Part model, mm, in its own coordinate system. Face numbers are marked on the shaded views. A direction names the side the tool comes from. Give positions to 0.01 mm unless a question says otherwise; leave off trailing zeros. Write each loop counter-clockwise with the first axis right and the second up, starting at its lowest first coordinate (ties: lowest second). Pieces come first, ordered by that corner, then holes. Notation, with made-up numbers: M -22.75,2 L 35.25,2 A22 cw 35.25,29 Z; hole C -40,4.25 d3. An arc over 180 degrees is marked long. Use a Markdown table: item, result.
```python
from build123d import *

# Parameters (mm, degrees)
SKETCH_W        = 160.02
SKETCH_H        = 160.02
PAD_DEPTH       = 5.08
SKETCH001_W     = 2.032
SKETCH001_H     = 160.02
PAD001_DEPTH    = 1.016
SKETCH002_W     = 160.02
SKETCH002_H     = 2.032
PAD002_DEPTH    = 1.016
SKETCH003_W     = 6.35
SKETCH003_H     = 12.7
PAD003_DEPTH    = 10.16
SKETCH004_R     = 2.032
POCKET_DEPTH    = 12.7
PAD004_DEPTH    = 160.02
PAD005_DEPTH    = 160.02
SKETCH007_R     = 5.2705
POCKET001_DEPTH = 7.366
SKETCH008_R     = 2.286
POCKET002_DEPTH = 12.7
SKETCH009_R     = 5.2705
POCKET003_DEPTH = 7.366
SKETCH010_R     = 2.286
POCKET004_DEPTH = 12.7
SKETCH011_R     = 5.2705
POCKET005_DEPTH = 7.366
SKETCH012_R     = 5.2705
POCKET006_DEPTH = 7.366
SKETCH013_R     = 2.286
POCKET007_DEPTH = 12.7
SKETCH014_R     = 2.286
POCKET008_DEPTH = 12.7
SKETCH015_W     = 6.35
SKETCH015_H     = 12.7
PAD006_DEPTH    = 10.16
SKETCH016_R     = 2.032
POCKET009_DEPTH = 12.7


with BuildPart() as part:
    # Sketch → Pad (new body)
    with BuildSketch(Plane.XY):
        with Locations((-8.701914, -21.351993)):
            Rectangle(SKETCH_W, SKETCH_H)
    extrude(amount=PAD_DEPTH)

    # Sketch001 (on Face6 of Pad) → Pad001 (join)
    with BuildSketch(Plane.XY.offset(5.08)):
        with Locations((-62.295914, -21.351993)):
            Rectangle(SKETCH001_W, SKETCH001_H)
        with Locations((44.892086, -21.351993)):
            Rectangle(SKETCH001_W, SKETCH001_H)
        with Locations((-13.527914, -21.351993)):
            Rectangle(SKETCH001_W, SKETCH001_H)
        with Locations((-3.875914, -21.351993)):
            Rectangle(SKETCH001_W, SKETCH001_H)
    extrude(amount=PAD001_DEPTH)

    # Sketch002 (on Face9 of Pad001) → Pad002 (join)
    with BuildSketch(Plane.XY.offset(5.08)):
        with Locations((-8.701914, 32.242007)):
            Rectangle(SKETCH002_W, SKETCH002_H)
        with Locations((-8.701914, -16.525993)):
            Rectangle(SKETCH002_W, SKETCH002_H)
        with Locations((-8.701914, -26.177993)):
            Rectangle(SKETCH002_W, SKETCH002_H)
        with Locations((-8.701914, -74.945993)):
            Rectangle(SKETCH002_W, SKETCH002_H)
    extrude(amount=PAD002_DEPTH)

    # Sketch003 (on Face164 of Pad002) → Pad003 (join)
    with BuildSketch(Plane.XY.offset(5.08)):
        with Locations((-56.961914, -44.211993)):
            Rectangle(SKETCH003_W, SKETCH003_H)
        with Locations((39.558086, -44.211993)):
            Rectangle(SKETCH003_W, SKETCH003_H)
    extrude(amount=PAD003_DEPTH)

    # Sketch004 (on Face174 of Pad003) → Pocket (cut)
    with BuildSketch(Plane.XZ.offset(50.561993)):
        with Locations((39.558086, 11.43)):
            Circle(SKETCH004_R)
        with Locations((-56.961914, 11.43)):
            Circle(SKETCH004_R)
    extrude(amount=-POCKET_DEPTH, mode=Mode.SUBTRACT)

    # Sketch005 (on Face14 of Pocket) → Pad004 (join)
    with BuildSketch(Plane.XZ.offset(101.361993)):
        Polygon((-88.711914, 5.08), (-88.711914, 22.86), (-84.901914, 22.86), (-76.011914, 8.89), (-76.011914, 5.08), align=None)
        Polygon((71.308086, 22.86), (67.498086, 22.86), (58.608086, 8.89), (58.608086, 5.08), (71.308086, 5.08), align=None)
    extrude(amount=-PAD004_DEPTH)

    # Sketch006 (on Face3 of Pad004) → Pad005 (join)
    with BuildSketch(Plane.YZ.offset(71.308086)):
        Polygon((-101.361993, 5.08), (-101.361993, 22.86), (-97.551993, 22.86), (-88.661993, 8.89), (-88.661993, 5.08), align=None)
        Polygon((58.658007, 5.08), (58.658007, 22.86), (54.848007, 22.86), (45.958007, 8.89), (45.958007, 5.08), align=None)
    extrude(amount=-PAD005_DEPTH)

    # Sketch007 (on Face66 of Pad005) → Pocket001 (cut)
    with BuildSketch(Plane(origin=(0, -88.661993, 0), x_dir=(-1, 0, 0), z_dir=(0, 1, 0))):
        with Locations((-39.558086, 15.24)):
            Circle(SKETCH007_R)
        with Locations((56.961914, 15.24)):
            Circle(SKETCH007_R)
        with Locations((8.701914, 15.24)):
            Circle(SKETCH007_R)
    extrude(amount=-POCKET001_DEPTH, mode=Mode.SUBTRACT)

    # Sketch008 (on Face66 of Pad005) → Pocket002 (cut)
    with BuildSketch(Plane(origin=(0, -88.661993, 0), x_dir=(-1, 0, 0), z_dir=(0, 1, 0))):
        with Locations((-39.558086, 15.24)):
            Circle(SKETCH008_R)
        with Locations((56.961914, 15.24)):
            Circle(SKETCH008_R)
        with Locations((8.701914, 15.24)):
            Circle(SKETCH008_R)
    extrude(amount=-POCKET002_DEPTH, mode=Mode.SUBTRACT)

    # Sketch009 (on Face53 of Pocket002) → Pocket003 (cut)
    with BuildSketch(Plane.YZ.offset(-76.011914)):
        with Locations((-69.611993, 15.24)):
            Circle(SKETCH009_R)
        with Locations((-21.351993, 15.24)):
            Circle(SKETCH009_R)
        with Locations((26.908007, 15.24)):
            Circle(SKETCH009_R)
    extrude(amount=-POCKET003_DEPTH, mode=Mode.SUBTRACT)

    # Sketch010 (on Face53 of Pocket003) → Pocket004 (cut)
    with BuildSketch(Plane.YZ.offset(-76.011914)):
        with Locations((-69.611993, 15.24)):
            Circle(SKETCH010_R)
        with Locations((-21.351993, 15.24)):
            Circle(SKETCH010_R)
        with Locations((26.908007, 15.24)):
            Circle(SKETCH010_R)
    extrude(amount=-POCKET004_DEPTH, mode=Mode.SUBTRACT)

    # Sketch011 (on Face54 of Pocket004) → Pocket005 (cut)
    with BuildSketch(Plane.XZ.offset(-45.958007)):
        with Locations((-56.961914, 15.24)):
            Circle(SKETCH011_R)
        with Locations((-8.701914, 15.24)):
            Circle(SKETCH011_R)
        with Locations((39.558086, 15.24)):
            Circle(SKETCH011_R)
    extrude(amount=-POCKET005_DEPTH, mode=Mode.SUBTRACT)

    # Sketch012 (on Face75 of Pocket005) → Pocket006 (cut)
    with BuildSketch(Plane(origin=(58.608086, 0, 0), x_dir=(0, -1, 0), z_dir=(-1, 0, 0))):
        with Locations((-26.908007, 15.24)):
            Circle(SKETCH012_R)
        with Locations((21.351993, 15.24)):
            Circle(SKETCH012_R)
        with Locations((69.611993, 15.24)):
            Circle(SKETCH012_R)
    extrude(amount=-POCKET006_DEPTH, mode=Mode.SUBTRACT)

    # Sketch013 (on Face75 of Pocket005) → Pocket007 (cut)
    with BuildSketch(Plane(origin=(58.608086, 0, 0), x_dir=(0, -1, 0), z_dir=(-1, 0, 0))):
        with Locations((-26.908007, 15.24)):
            Circle(SKETCH013_R)
        with Locations((21.351993, 15.24)):
            Circle(SKETCH013_R)
        with Locations((69.611993, 15.24)):
            Circle(SKETCH013_R)
    extrude(amount=-POCKET007_DEPTH, mode=Mode.SUBTRACT)

    # Sketch014 (on Face54 of Pocket004) → Pocket008 (cut)
    with BuildSketch(Plane.XZ.offset(-45.958007)):
        with Locations((-56.961914, 15.24)):
            Circle(SKETCH014_R)
        with Locations((-8.701914, 15.24)):
            Circle(SKETCH014_R)
        with Locations((39.558086, 15.24)):
            Circle(SKETCH014_R)
    extrude(amount=-POCKET008_DEPTH, mode=Mode.SUBTRACT)

    # Sketch015 (on Face164 of Pad002) → Pad006 (join)
    with BuildSketch(Plane.XY.offset(5.08)):
        with Locations((-56.961914, 1.508007)):
            Rectangle(SKETCH015_W, SKETCH015_H)
        with Locations((39.558086, 1.508007)):
            Rectangle(SKETCH015_W, SKETCH015_H)
    extrude(amount=PAD006_DEPTH)

    # Sketch016 (on Face254 of Pad006) → Pocket009 (cut)
    with BuildSketch(Plane(origin=(0, 7.858007, 0), x_dir=(-1, 0, 0), z_dir=(0, 1, 0))):
        with Locations((56.961914, 11.176)):
            Circle(SKETCH016_R)
        with Locations((-39.558086, 11.176)):
            Circle(SKETCH016_R)
    extrude(amount=-POCKET009_DEPTH, mode=Mode.SUBTRACT)


solid = part.part
```
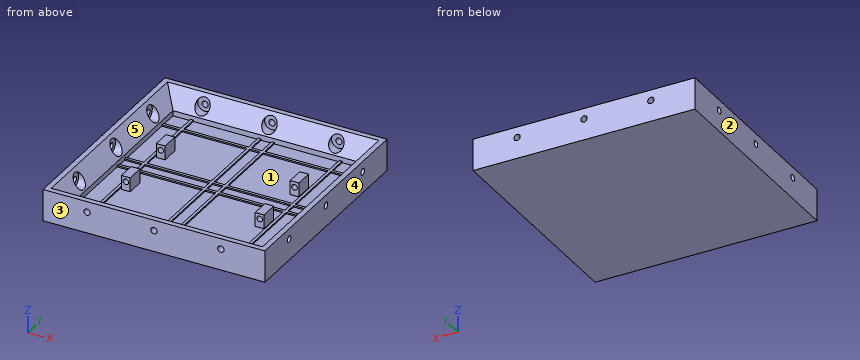
1. Drop flat-ended pins along their axis: P1, Ø6, axis at x = -9, y = -20, coming from the +Z side; P2, Ø7, axis at x = -57.5, y = -45, coming from the +Z side; P3, Ø2.5, axis at x = -9, y = -79.5, coming from the +Z side. Give the stop position or say it passes through.
Findings below:
| item | result |
|---|---|
| P1 | z = 6.1 |
| P2 | z = 15.24 |
| P3 | z = 5.08 |
2. Two-plate mould, pull along Y, no slides. Class the marked faces 1, 2 and 3: released by +Y, released by -Y, zero draft, split by the parting line, or undercut.
Findings below:
| item | result |
|---|---|
| face 1 | undercut |
| face 2 | zero draft |
| face 3 | released by -Y |
3. Cut at A-A, the plane y = -85. Give the cut face in (x, z).
Findings below:
| item | result |
|---|---|
| outline | M -88.71,0 L 71.31,0 L 71.31,22.86 L 67.5,22.86 L 58.61,8.89 L 58.61,5.08 L 45.91,5.08 L 45.91,6.1 L 43.88,6.1 L 43.88,5.08 L -2.86,5.08 L -2.86,6.1 L -4.89,6.1 L -4.89,5.08 L -12.51,5.08 L -12.51,6.1 L -14.54,6.1 L -14.54,5.08 L -61.28,5.08 L -61.28,6.1 L -63.31,6.1 L -63.31,5.08 L -76.01,5.08 L -76.01,8.89 L -84.9,22.86 L -88.71,22.86 Z |
4. Drill centre lines: L1, parallel to Y at x = 41, z = 18.5; L2, parallel to Y at x = 54.5, z = 8; L3, parallel to X at y = 52.25, z = 15.24. Where is each one in solid material? Low to high.
Findings below:
| item | result |
|---|---|
| L1 | -101.36 to -96.03, 53.32 to 58.66 |
| L2 | -101.36 to -88.66, 45.96 to 58.66 |
| L3 | -88.71 to -62.23, -51.69 to -13.97, -3.43 to 34.29, 44.83 to 71.31 |
5. Cut at B-B, the plane x = -25.5. Give the cut face in (y, z), then the cut area to 3 significant figures.
Findings below:
| item | result |
|---|---|
| outline | M -101.36,0 L 58.66,0 L 58.66,22.86 L 54.85,22.86 L 45.96,8.89 L 45.96,5.08 L 33.26,5.08 L 33.26,6.1 L 31.23,6.1 L 31.23,5.08 L -15.51,5.08 L -15.51,6.1 L -17.54,6.1 L -17.54,5.08 L -25.16,5.08 L -25.16,6.1 L -27.19,6.1 L -27.19,5.08 L -73.93,5.08 L -73.93,6.1 L -75.96,6.1 L -75.96,5.08 L -88.66,5.08 L -88.66,8.89 L -97.55,22.86 L -101.36,22.86 Z |
| area | 1,150 mm2 |
6. Tool access for the marked faces 4 and 5: list every direction of +Z, -Z, +X, -X, +Y, -Y with a clear straight run to the whole face (end or side of a thin tool).
Findings below:
| item | result |
|---|---|
| face 4 | +Z, -Z, +X, +Y, -Y |
| face 5 | +Z |
